Can you work these out from the model? Positions are in its coordinate system, mm. Round coordinates to 2 decimals unless told otherwise and drop trailing zeros. Write each loop counter-clockwise with the first axis right and the second up, starting at its lowest first coordinate (ties: lowest second). Pieces come first, ordered by that corner, then holes. Notation, with made-up numbers: M 82,-11.75 L 132,-11.75 A23 ccw 132,8.25 Z; hole C 25.5,21 d7. An arc over 180 degrees is marked long. Answer as a JSON object with one key per item and string values. Group by question number.
1) Please list where these lines run through material, in increasing order: L1, parallel to Y at x = 24.5, z = 19.5; L2, parallel to Y at x = -4.5, z = 2.5; L3, parallel to X at y = -5.5, z = 10. Write a range as [from, to].
2) I'm going to push flat-ended pins straight in: pin 1 Ø3 at (y, z) = (27.5, 50) entering from -X; pin 2 Ø1.5 at (y, z) = (-21.5, 48) entering from -X; pin 3 Ø3 at (x, z) = (20.5, 22.5) entering from -Y; pin 4 Ø4 at (x, y) = (-13, 40) entering from -Z. Where does each tip first touch, or does it pass through?
3) Suppose I cut it at B-B, the plane x = -30. Write out the boundary of the cut face in (y, z), and give its area (3 significant figures).
4) Suppose I cut it at A-A, the plane x = -13.5. Write out the boundary of the cut face in (y, z), and give its area (4 significant figures).
from build123d import *

# Parameters (mm, degrees)
F1_DEPTH = 58.42
F2_R     = 15.24
F3_R     = 6.8301694269
F4_DEPTH = 30.48


with BuildPart() as f1:
    # F0 (on Top) → F1 (new body)
    with BuildSketch(Plane.XY):
        with BuildLine():
            ThreePointArc((-22.9468365368, 28.7332625584), (-15.943079518, -33.1357193942), (36.7716967829, 0))
            ThreePointArc((36.7716967829, 0), (29.0432904816, 22.553158588), (9.1066714076, 35.6262013154))
            ThreePointArc((9.1066714076, 35.6262013154), (-7.7308275028, 35.9498538302), (-22.9468365368, 28.7332625584))
        make_face()
        with BuildLine():
            ThreePointArc((-22.9468365368, 28.7332625584), (-7.7308275028, 35.9498538302), (9.1066714076, 35.6262013154))
            ThreePointArc((9.1066714076, 35.6262013154), (-11.3815660909, 52.926499418), (-22.9468365368, 28.7332625584))
        make_face()
    extrude(amount=F1_DEPTH)

    # F2
    f2_edges = [f1.edges().sort_by_distance(p)[0] for p in [
        (9.106671, 35.626201, 29.21),
        (-22.946837, 28.733263, 29.21),
    ]]
    fillet(f2_edges, radius=F2_R)

    # F3 (on face) → F4 (join)
    with BuildSketch(Plane.XY.offset(58.42)):
        with Locations((-1.7507391749, 3.4323732834)):
            Circle(F3_R)
    extrude(amount=-F4_DEPTH)


solid = f1.part
Results:
{
 "1": {"L1": "[-27.42, 27.42]", "L2": "[-36.5, 52.98]", "L3": "[-36.36, 36.36]"},
 "2": {"pin 1": "x = -26.55", "pin 2": "x = -30.36", "pin 3": "y = -31.48", "pin 4": "z = 0"},
 "3": {"outline": "M -21.26,0 L 21.26,0 L 21.26,58.42 L -21.26,58.42 Z", "area": "2,480 mm^2"},
 "4": {"outline": "M -34.2,0 L 52.32,0 L 52.32,58.42 L -34.2,58.42 Z", "area": "5,055 mm^2"}
}
